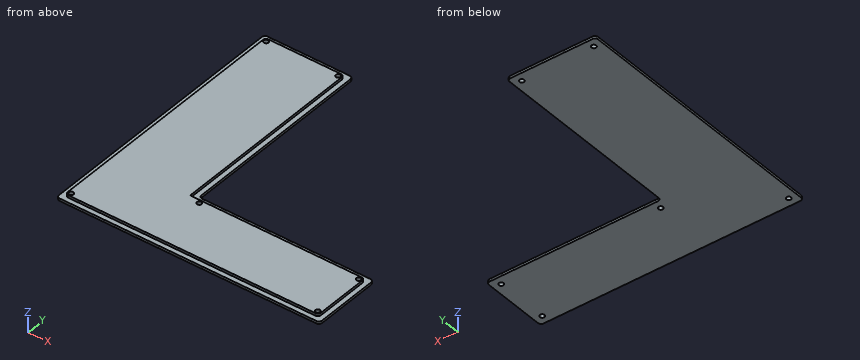
Autodesk Inventor part; units mm, degrees
ref_plane "YZ Plane" through (0, 0, 0) normal (1, 0, 0) x (0, 1, 0)
ref_plane "XZ Plane" through (0, 0, 0) normal (0, 1, 0) x (-1, 0, 0)
ref_plane "XY Plane" through (0, 0, 0) normal (0, 0, 1) x (1, 0, 0)
sketch "Sketch1" plane through (0, 0, 0) normal (0, 0, 1) x (1, 0, 0)
  line L0 (0, 0) -> (3.175, 0)
  line L1 (3.175, 0) -> (53.975, 0)
  line L2 (53.975, 0) -> (57.15, 0)
  line L3 (57.15, 0) -> (57.15, -127)
  line L4 (57.15, -127) -> (111.887, -127)
  line L5 (111.887, -127) -> (169.799, -127)
  line L6 (169.799, -127) -> (169.799, -130.175)
  line L7 (169.799, -130.175) -> (169.799, -168.275)
  line L8 (169.799, -168.275) -> (169.799, -171.45)
  line L9 (169.799, -171.45) -> (57.15, -171.45)
  line L10 (57.15, -171.45) -> (0, -171.45)
  line L11 (0, -171.45) -> (0, 0)
  dimension "d0" = 3.175
  dimension "d1" = 50.8
  dimension "d2" = 3.175
  dimension "d3" = 127
  dimension "d4" = 54.737
  dimension "d5" = 57.912
  dimension "d6" = 3.175
  dimension "d7" = 38.1
  dimension "d8" = 3.175
extrude "Extrusion1" add sketch "Sketch1" along normal blind 1.5875
sketch "Sketch2" plane through (0, 0, 1.5875) normal (0, 0, 1) x (1, 0, 0)
  line L0 (57.15, 0) -> (0, 0)
  line L1 (0, 0) -> (0, -171.45)
  line L2 (0, -171.45) -> (169.799, -171.45)
  line L3 (169.799, -171.45) -> (169.799, -127)
  line L4 (169.799, -127) -> (57.15, -127)
  line L5 (3.175, -3.175) -> (3.175, -168.275)
  line L6 (3.175, -168.275) -> (166.624, -168.275)
  line L7 (166.624, -168.275) -> (166.624, -130.175)
  line L8 (166.624, -130.175) -> (53.975, -130.175)
  line L9 (53.975, -130.175) -> (53.975, -3.175)
  line L10 (3.175, -3.175) -> (53.975, -3.175)
extrude "Extrusion2" add sketch "Sketch2" along normal blind 1.5875
sketch "Sketch3" plane through (0, 0, 0) normal (0, 0, -1) x (-1, 0, 0)
  line L0 (-169.799, -127) -> (-57.15, -127)
  line L1 (-57.15, -127) -> (-57.15, -130.175)
  line L2 (-53.975, -130.175) -> (-166.624, -130.175)
  line L3 (-57.15, -130.175) -> (-61.55, -130.175)
  line L4 (-61.55, -130.175) -> (-61.55, -132.325)
  line L5 (-166.624, -168.275) -> (-166.624, -130.175)
  line L6 (-166.624, -130.175) -> (-164.474, -130.175)
  line L7 (-164.474, -130.175) -> (-164.474, -132.325)
  line L8 (-166.624, -168.275) -> (-3.175, -168.275)
  line L9 (-166.624, -168.275) -> (-164.474, -168.275)
  line L10 (-164.474, -168.275) -> (-164.474, -166.125)
  line L11 (-3.175, -168.275) -> (-3.175, -3.175)
  line L12 (-3.175, -168.275) -> (-5.325, -168.275)
  line L13 (-5.325, -168.275) -> (-5.325, -166.125)
  line L14 (-3.175, -3.175) -> (-5.325, -3.175)
  line L15 (-3.175, -3.175) -> (-53.975, -3.175)
  line L16 (-5.325, -3.175) -> (-5.325, -5.325)
  line L17 (-53.975, -3.175) -> (-51.825, -3.175)
  line L18 (-51.825, -3.175) -> (-51.825, -5.325)
  point P0 (0, 0)
  dimension "d23" = 4.4
  dimension "d24" = 2.15
  dimension "d25" = 270
  dimension "d26" = 2.15
  dimension "d27" = 2.15
  dimension "d28" = 2.15
  dimension "d29" = 2.15
  dimension "d30" = 2.15
  dimension "d31" = 2.15
  dimension "d32" = 2.15
  dimension "d33" = 2.15
  dimension "d34" = 2.15
hole "Hole1" at (51.825, -5.325, 0) at (5.325, -5.325, 0) at (61.55, -132.325, 0) at (5.325, -166.125, 0) at (164.474, -166.125, 0) at (164.474, -132.325, 0) direction (0, 0, 1) diameter 3 depth 3.175
fillet "Fillet1" radius 2 11 edges at (169.799, -127, 0.7937) (166.624, -130.175, 2.3812) (166.624, -168.275, 2.3812) (169.799, -171.45, 0.7937) (57.15, -127, 0.7937) (3.175, -168.275, 2.3812) (0, -171.45, 0.7937) (57.15, 0, 0.7937) (53.975, -3.175, 2.3812) (3.175, -3.175, 2.3812) (0, 0, 0.7937)
properties part number "Main Body Lid Backwards"
The model under review builds one solid part; all positions refer to its coordinate system, in mm. Round coordinates to 2 decimals unless told otherwise and drop trailing zeros. Order: outer loops, then holes, each group sorted by start corner. A loop starts at its lowest first (then second) coordinate and runs counter-clockwise, first axis right, second up. Notation, with made-up numbers: (52, 83.5) -> (70, 83.5) arc R16 ccw to (70, 90.5) -> close; hole circle Ø4 at (86, 22). An arc over 180 degrees is marked (long way). Use CSV: the item, a comma, the result in double quotes. Start each with the question number.
(1) Consider section C-C on y = -153. Write out the cut boundary in (x, z) (1 decimal), and give its area (3 significant figures).
(2) Wall thickness on probe 1 along Y at (x, z) = (61.55, 1.65) (3 decimals); probe 2 along X at (y, z) = (-55.5, 1.8) (3 decimals); probe 3 along Y at (x, z) = (153.5, 2.6) (3 decimals): over which ranges is each line inside the solid? List them lowest first. Write a range as from..to.
(3) Consider section B-B on z = 1. Write out the cut boundary in (x, y) (3 decimals).
(4) Insertion check: pin 1 (0.5 mm diameter, centred on x = 27.5, z = 2.5, fed in from +Y) (3 decimals); pin 2 (0.5 mm diameter, centred on y = -54, z = 2, fed in from +X) (3 decimals); pin 3 (1.3 mm diameter, centred on x = 95, z = 1, fed in from +Y). Each pin has a flat end and moves straight along its axis. Give the tip position at first contact, or say it passes through.
Responses:
1,outline,"(0, 0) -> (169.8, 0) -> (169.8, 1.6) -> (166.6, 1.6) -> (166.6, 3.2) -> (3.2, 3.2) -> (3.2, 1.6) -> (0, 1.6) -> close"
1,area,"529 mm²"
2,probe 1,"-168.275..-133.825, -130.825..-130.175"
2,probe 2,"3.175..53.975"
2,probe 3,"-168.275..-130.175"
3,outline,"(0, -169.45) arc R2 ccw to (2, -171.45) -> (167.799, -171.45) arc R2 ccw to (169.799, -169.45) -> (169.799, -129) arc R2 ccw to (167.799, -127) -> (59.15, -127) arc R2 cw to (57.15, -125) -> (57.15, -2) arc R2 ccw to (55.15, 0) -> (2, 0) arc R2 ccw to (0, -2) -> close; hole circle Ø3 at (5.325, -166.125); hole circle Ø3 at (5.325, -5.325); hole circle Ø3 at (51.825, -5.325); hole circle Ø3 at (61.55, -132.325); hole circle Ø3 at (164.474, -166.125); hole circle Ø3 at (164.474, -132.325)"
4,pin 1,"y = -3.175"
4,pin 2,"x = 53.975"
4,pin 3,"y = -127"
